```python
from build123d import *

# Parameters (mm, degrees)
BOSS_EXTRUDE1_DEPTH = 5
CUT_EXTRUDE1_DEPTH  = 10


with BuildPart() as part:
    # Sketch1 → Boss-Extrude1 (new, symmetric)
    with BuildSketch(Plane.XY):
        Polygon((0, 0), (20, 20), (-20, 20), align=None)
    extrude(amount=BOSS_EXTRUDE1_DEPTH, both=True)

    # Sketch2 → Cut-Extrude1 (cut)
    with BuildSketch(Plane.XY.offset(5)):
        Polygon((0, 2.828427125), (-17.171572875, 20), (17.171572875, 20), align=None)
    extrude(amount=-CUT_EXTRUDE1_DEPTH, mode=Mode.SUBTRACT)


solid = part.part
```
Source: CAD feature listing. Evaluate the final solid. Frame: model axes, mm. A direction names the side the tool comes from. Coordinates: 2 decimals unless noted, no trailing zeros. Loops run counter-clockwise (first coordinate to the right, second up) from the corner with the lowest first, then second, coordinate; pieces in that order, holes last. Notation, with made-up numbers: (-17.75, 37.25) - (39.25, 37.25) arc R7 cw to (39.25, 46.25) - close; hole circle Ø3 at (29, 25.25). An arc over 180 degrees is marked (long way). Answer as CSV lines item,"result".
1. Section B-B (z = 1.75). Return loops of the section in (x, y).
Established:
outline,"(-20, 20) - (0, 0) - (20, 20) - (17.17, 20) - (0, 2.83) - (-17.17, 20) - close"
2. Ray query, line 1 (X direction, y = 18.5, z = 4); line 2 (X direction, y = 5.5, z = 0.5); line 3 (Y direction, x = -9, z = 3.25). Return the intervals inside material, ascending.
Established:
line 1,"x = -18.5 to -15.67, 15.67 to 18.5"
line 2,"x = -5.5 to -2.67, 2.67 to 5.5"
line 3,"y = 9 to 11.83"
3. Reachability of faces 1 (the flat face through (8.706, 11.534, 0.07)), 2 (the flat face through (-3.1, 5.6, -5)) from +Z, -Z, +X, -X, +Y, -Y: full face, straight path, thin tool, end or side. Return the list, or none.
Established:
face 1,"+Z, -Z, +Y"
face 2,"-Z, +X, -X, +Y, -Y"
4. Section A-A (y = 19). Return loops of the section in (x, z).
Established:
outline,"(-19, -5) - (-16.17, -5) - (-16.17, 5) - (-19, 5) - close; (16.17, -5) - (19, -5) - (19, 5) - (16.17, 5) - close"
5. Mould query, pull axis X, two halves, no side actions, for faces 3 (the flat face through (-8.466, 11.294, 0.07)), 4 (the flat face through (-10, 10, 0)), 5 (the flat face through (10, 10, 0)). Classes: released by +X, released by -X, zero draft, split by the parting line, or undercut.
Established:
face 3,"undercut"
face 4,"released by -X"
face 5,"released by +X"
6. Section C-C (x = -1). Return loops of the section in (y, z), then the cut area to 3 significant figures.
Established:
outline,"(1, -5) - (3.83, -5) - (3.83, 5) - (1, 5) - close"
area,"28.3 mm2"
7. Contact query for flat-ended pins moving along their axis: pin 1 (5 mm diameter, centred on x = 1.5, z = 2, fed in from +Y); pin 2 (12 mm diameter, centred on x = 3.5, y = 10.5, fed in from -Z); pin 3 (3 mm diameter, centred on x = 15, y = 11, fed in from +Z); pin 4 (6 mm diameter, centred on x = 6.5, z = 4, fed in from +Y). Output: stop coordinate, or through.
Established:
pin 1,"stops at y = 6.83"
pin 2,"stops at z = -5"
pin 3,"passes through"
pin 4,"stops at y = 12.33"
